Build history of the part. All positions in model axes, mm. A direction names the side the tool comes from. Round coordinates to 2 decimals unless told otherwise and drop trailing zeros. Loops run counter-clockwise (first coordinate to the right, second up) from the corner with the lowest first, then second, coordinate; pieces in that order, holes last. Notation, with made-up numbers: (29, -24.5) - (56, -24.5) arc R14 cw to (56, -5.5) - close; hole circle Ø2 at (-27.75, 62). An arc over 180 degrees is marked (long way). Use a Markdown table: item, result.
from build123d import *

# Parameters (mm, degrees)
F0_R     = 1.75
F1_DEPTH = 2
F2_R     = 1.99999


# Not quite as in the source:
# - a fillet or chamfer is up to 0.001 mm smaller than in the source, because OpenCascade refuses the exact size


with BuildPart() as f1:
    # F0 (on Top) → F1 (new body)
    with BuildSketch(Plane.XY):
        with BuildLine():
            Line((0, 22), (0, 0))
            ThreePointArc((0, 0), (10.8792490031, 0.5215994991), (21.6586962342, 2.0816130564))
            ThreePointArc((21.6586962342, 2.0816130564), (49.1649189112, 6.6602813892), (77, 8.3230352611))
            ThreePointArc((77, 8.3230352611), (77.9999938672, 8.3281723489), (79, 8.3295355292))
            ThreePointArc((79, 8.3295355292), (81.0000609284, 8.3209395881), (83, 8.2972474438))
            ThreePointArc((83, 8.2972474438), (84.0000366078, 8.2797378058), (85, 8.2584535703))
            Line((85, 8.2584535703), (85, 13.7415464297))
            ThreePointArc((85, 13.7415464297), (84.0000366078, 13.7202621942), (83, 13.7027525562))
            ThreePointArc((83, 13.7027525562), (81.0000609284, 13.6790604119), (79, 13.6704644708))
            ThreePointArc((79, 13.6704644708), (77.9999938672, 13.6718276511), (77, 13.6769647389))
            ThreePointArc((77, 13.6769647389), (49.1649189112, 15.3397186108), (21.6586962342, 19.9183869436))
            ThreePointArc((21.6586962342, 19.9183869436), (10.8792490031, 21.4784005009), (0, 22))
        make_face()
        with Locations((3, 4.3338485993)):
            Circle(F0_R, mode=Mode.SUBTRACT)
        with Locations((3, 17.3932574689)):
            Circle(F0_R, mode=Mode.SUBTRACT)
        with BuildLine():
            ThreePointArc((79, 8.3295355292), (77.9999938672, 8.3281723489), (77, 8.3230352611))
            Line((77, 8.3230352611), (77, 5.2972474438))
            Line((77, 5.2972474438), (79, 5.2972474438))
            Line((79, 5.2972474438), (79, 8.3295355292))
        make_face()
        with BuildLine():
            Line((83, 5.2972474438), (85, 5.2972474438))
            Line((85, 5.2972474438), (85, 8.2584535703))
            ThreePointArc((85, 8.2584535703), (84.0000366078, 8.2797378058), (83, 8.2972474438))
            Line((83, 8.2972474438), (83, 5.2972474438))
        make_face()
        with BuildLine():
            Line((77, 16.7027525562), (77, 13.6769647389))
            ThreePointArc((77, 13.6769647389), (77.9999938672, 13.6718276511), (79, 13.6704644708))
            Line((79, 13.6704644708), (79, 16.7027525562))
            Line((79, 16.7027525562), (77, 16.7027525562))
        make_face()
        with BuildLine():
            Line((85, 13.7415464297), (85, 16.7027525562))
            Line((85, 16.7027525562), (83, 16.7027525562))
            Line((83, 16.7027525562), (83, 13.7027525562))
            ThreePointArc((83, 13.7027525562), (84.0000366078, 13.7202621942), (85, 13.7415464297))
        make_face()
    extrude(amount=F1_DEPTH)

    # F2 (radius 2 in the source; OpenCascade refuses exactly that, so slightly less here)
    f2_edges = [f1.edges().sort_by_distance(p)[0] for p in [
        (0, 0, 1),
        (0, 22, 1),
        (85, 5.297247, 1),
        (85, 16.702753, 1),
        (77, 8.323035, 1),
        (77, 13.676965, 1),
    ]]
    fillet(f2_edges, radius=F2_R)


solid = f1.part
Q1. Which spindle directions (+Z, -Z, +X, -X, +Y, -Y) get a long thin tool onto all of the face, cutting with end or side? Do faces 1 (the face through (76.39, 7.74, 1.01)), 2 (the face through (78, 5.297, 1)), 3 (the face through (78, 16.703, 1)), 4 (the face through (79, 15, 1)). Say none if no direction does.
Results found:
| item | result |
|---|---|
| face 1 | +Z, -Z, -Y |
| face 2 | +Z, -Z, +X, -Y |
| face 3 | +Z, -Z, +X, +Y |
| face 4 | +Z, -Z, +Y |
Q2. Cut at C-C, the plane x = 14.5. List the corners of the cut face in (y, z).
Results found:
| item | result |
|---|---|
| outline | (0.93, 0) - (21.07, 0) - (21.07, 2) - (0.93, 2) - close |
Q3. Cut at D-D, the plane x = 46.5. List the corners of the cut face in (y, z), plus the area to 3 significant figures.
Results found:
| item | result |
|---|---|
| outline | (6.35, 0) - (15.65, 0) - (15.65, 2) - (6.35, 2) - close |
| area | 18.6 mm2 |
Q4. Cut at A-A, the plane x = 3. List the corners of the cut face in (y, z).
Results found:
| item | result |
|---|---|
| outline | (0.04, 0) - (2.58, 0) - (2.58, 2) - (0.04, 2) - close; (6.08, 0) - (15.64, 0) - (15.64, 2) - (6.08, 2) - close; (19.14, 0) - (21.96, 0) - (21.96, 2) - (19.14, 2) - close |
Q5. Cut at B-B, the plane z = 1.55. Count the separate pieces of the cut face and the enclosed holes in it, plus the area to 3 significant figures.
Results found:
| item | result |
|---|---|
| separate pieces | 1 |
| enclosed holes | 2 |
| area | 1,030 mm2 |
Q6. Drop flat-ended pins along their axis: pin 1 (1 mm diameter, centred on x = 78.5, z = 1, fed in from -Y); pin 2 (0.6 mm diameter, centred on x = 78, z = 1.5, fed in from +Y). Give the stop position or say it passes through.
Results found:
| item | result |
|---|---|
| pin 1 | stops at y = 5.3 |
| pin 2 | stops at y = 16.7 |
Q7. Probe line 1 (Y direction, x = 3, z = 1.4); line 2 (Y direction, x = 77.5, z = 1.45); line 3 (Y direction, x = 49.5, z = 1.65). List the from-to ranges inside material, lowest first.
Results found:
| item | result |
|---|---|
| line 1 | y = 0.04 to 2.58, 6.08 to 15.64, 19.14 to 21.96 |
| line 2 | y = 5.3 to 16.7 |
| line 3 | y = 6.7 to 15.3 |
Q8. Pull direction X, two halves, no side cores. Call faces 5 (the face through (84.4, 5.87, 1.01)), 6 (the face through (48.531, 15.412, 0.986)), 7 (the face through (32, 11, 0)): pulls with the +X half, pulls with the -X half, needs draft (parallel to the pull), parting line crosses it, or undercut.
Results found:
| item | result |
|---|---|
| face 5 | pulls with the +X half |
| face 6 | undercut |
| face 7 | needs draft |
